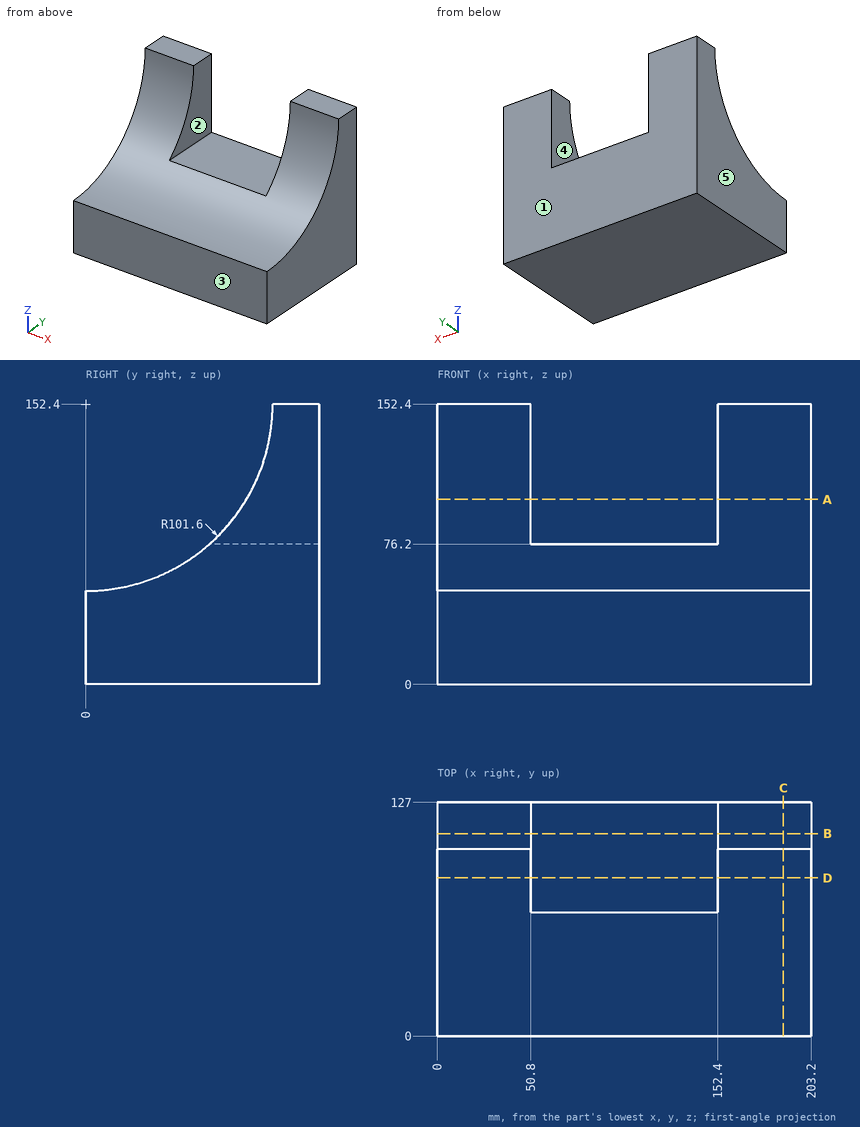
Source: three-view drawing plus pictorial views. Frame: mm from the lowest corner of the part. A direction names the side the tool comes from. Give positions to 0.01 mm unless a question says otherwise; leave off trailing zeros. Write each loop counter-clockwise with the first axis right and the second up, starting at its lowest first coordinate (ties: lowest second). Pieces come first, ordered by that corner, then holes.
(1) Cut plane B-B, the plane y = 110. Return loops of the section in (x, z).
(2) First-contact query: P1, Ø12, axis at x = 97.5, y = 40.5, coming from the -Z side; P2, Ø6, axis at x = 99, y = 94, coming from the +Z side. Flat tips, straight axial feed; report the tip coordinate or a pass-through.
(3) Mould query, pull axis X, two halves, no side actions, for the marked faces 3, 4 and 5. Classes: released by +X, released by -X, zero draft, split by the parting line, or undercut.
(4) Ray query, line 1 (X direction, y = 117, z = 145); line 2 (Z direction, x = 84.5, y = 73.5); line 3 (Z direction, x = 46, y = 62). Return the intervals inside material, ascending.
(5) Access query for the marked faces 1 and 2. Directions: +Z, -Z, +X, -X, +Y, -Y. A direction counts if a zero-diameter tool reaches every point of the face in a straight line with its end or side. Return the directions, or none.
(6) Cut plane D-D, the plane y = 86. Return loops of the section in (x, z), then the cut area to 3 significant figures.
(7) Cut plane C-C, the plane x = 188. Return loops of the section in (y, z), then the cut area to 3 significant figures.
(8) Cut plane A-A, the plane z = 100.5. Return loops of the section in (x, y).
Values follow:
1. outline: (0, 0) - (203.2, 0) - (203.2, 152.4) - (152.4, 152.4) - (152.4, 76.2) - (50.8, 76.2) - (50.8, 152.4) - (0, 152.4) - close
2. P1: stops at z = 0
2. P2: stops at z = 76.2
3. face 3: zero draft
3. face 4: undercut
3. face 5: released by -X
4. line 1: x = 0 to 50.8, 152.4 to 203.2
4. line 2: z = 0 to 76.2
4. line 3: z = 0 to 71.91
5. face 1: +Z, -Z, +X, -X, +Y
5. face 2: +Z, +Y, -Y
6. outline: (0, 0) - (203.2, 0) - (203.2, 98.3) - (152.4, 98.3) - (152.4, 76.2) - (50.8, 76.2) - (50.8, 98.3) - (0, 98.3) - close
6. area: 17,700 mm2
7. outline: (0, 0) - (127, 0) - (127, 152.4) - (101.6, 152.4) arc R101.6 cw to (0, 50.8) - close
7. area: 11,200 mm2
8. outline: (0, 87.34) - (50.8, 87.34) - (50.8, 127) - (0, 127) - close; (152.4, 87.34) - (203.2, 87.34) - (203.2, 127) - (152.4, 127) - close
